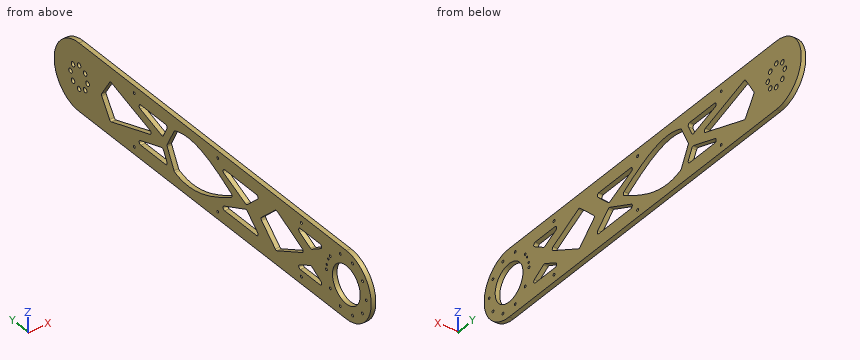
from build123d import *

# Parameters (mm, degrees)
SKETCH1_R           = 3.3
SKETCH1_R_2         = 1.7
SKETCH1_R_3         = 26
BOSS_EXTRUDE1_DEPTH = 6.35
CUT_EXTRUDE1_DEPTH  = 549.511460682
FILLET1_R           = 3
SKETCH4_R           = 1.75
CUT_EXTRUDE2_DEPTH  = 549.511460792
SKETCH5_R           = 1.2
CUT_EXTRUDE4_DEPTH  = 549.511460792


with BuildPart() as part:
    # Sketch1 → Boss-Extrude1 (new body)
    with BuildSketch(Plane(origin=(0, 0, 0), x_dir=(0, -1, 0), z_dir=(1, 0, 0))):
        with BuildLine():
            Line((0, 46.5), (500, 46.5))
            ThreePointArc((500, 46.5), (546.5, 0), (500, -46.5))
            Line((500, -46.5), (0, -46.5))
            ThreePointArc((0, -46.5), (-46.5, 0), (0, 46.5))
        make_face()
        with Locations(Location((-16, 0, 0), (0, 0, 90))):
            Circle(SKETCH1_R, mode=Mode.SUBTRACT)
        with Locations(Location((-11.313708499, 11.313708499, 0), (0, 0, 90))):
            Circle(SKETCH1_R, mode=Mode.SUBTRACT)
        with Locations(Location((0, 16, 0), (0, 0, 90))):
            Circle(SKETCH1_R, mode=Mode.SUBTRACT)
        with Locations(Location((11.313708499, 11.313708499, 0), (0, 0, 90))):
            Circle(SKETCH1_R, mode=Mode.SUBTRACT)
        with Locations(Location((16, 0, 0), (0, 0, 90))):
            Circle(SKETCH1_R, mode=Mode.SUBTRACT)
        with Locations(Location((11.313708499, -11.313708499, 0), (0, 0, 90))):
            Circle(SKETCH1_R, mode=Mode.SUBTRACT)
        with Locations(Location((537.25, 0, 0), (0, 0, 90))):
            Circle(SKETCH1_R_2, mode=Mode.SUBTRACT)
        with Locations(Location((530.13588304, -21.895000648, 0), (0, 0, 90))):
            Circle(SKETCH1_R_2, mode=Mode.SUBTRACT)
        with Locations(Location((511.51088304, -35.426855232, 0), (0, 0, 90))):
            Circle(SKETCH1_R_2, mode=Mode.SUBTRACT)
        with Locations(Location((488.48911696, -35.426855232, 0), (0, 0, 90))):
            Circle(SKETCH1_R_2, mode=Mode.SUBTRACT)
        with Locations(Location((469.86411696, -21.895000648, 0), (0, 0, 90))):
            Circle(SKETCH1_R_2, mode=Mode.SUBTRACT)
        with Locations(Location((462.75, 0, 0), (0, 0, 90))):
            Circle(SKETCH1_R_2, mode=Mode.SUBTRACT)
        with Locations(Location((469.86411696, 21.895000648, 0), (0, 0, 90))):
            Circle(SKETCH1_R_2, mode=Mode.SUBTRACT)
        with Locations(Location((488.48911696, 35.426855232, 0), (0, 0, 90))):
            Circle(SKETCH1_R_2, mode=Mode.SUBTRACT)
        with Locations(Location((511.51088304, 35.426855232, 0), (0, 0, 90))):
            Circle(SKETCH1_R_2, mode=Mode.SUBTRACT)
        with Locations(Location((530.13588304, 21.895000648, 0), (0, 0, 90))):
            Circle(SKETCH1_R_2, mode=Mode.SUBTRACT)
        with Locations(Location((500, 0, 0), (0, 0, 90))):
            Circle(SKETCH1_R_3, mode=Mode.SUBTRACT)
        with Locations(Location((0, -16, 0), (0, 0, 90))):
            Circle(SKETCH1_R, mode=Mode.SUBTRACT)
        with Locations(Location((-11.313708499, -11.313708499, 0), (0, 0, 90))):
            Circle(SKETCH1_R, mode=Mode.SUBTRACT)
    extrude(amount=BOSS_EXTRUDE1_DEPTH)

    # Sketch3 → Cut-Extrude1 (cut, through all)
    with BuildSketch(Plane(origin=(6.35, 0, 0), x_dir=(0, 0, -1), z_dir=(1, 0, 0))):
        Polygon((0, -422.848022722), (27.858212922, -368.632839363), (0, -339.139268075), (-27.858212922, -368.632839363), align=None)
        Polygon((0, -41.368651369), (-27.312924288, -58.435222232), (0, -141.248998295), (27.312924288, -58.435222232), align=None)
        Polygon((3, -313.189087212), (27.858212922, -339.506549748), (27.858212922, -258.646044282), align=None)
        Polygon((-27.858212922, -339.506549748), (-27.858212922, -258.646044282), (-3, -313.189087212), align=None)
        Polygon((-27.858212922, -401.452857349), (-11, -434.260816252), (-27.858212922, -461.481824785), align=None)
        Polygon((11, -434.260816252), (27.858212922, -461.481824785), (27.858212922, -401.452857349), align=None)
        with BuildLine():
            Line((0, -164.248853344), (-27.858212922, -178.200474573))
            add(Edge.make_bspline(
                [(-27.858212922, -178.200474573), (-43.7790539, -216.093343216), (-18.61661693, -258.276071598), (0, -289.085024731)],
                knots=[0, 0, 0, 0, 1, 1, 1, 1], degree=3))
            add(Edge.make_bspline(
                [(27.858212922, -178.200474573), (43.7790539, -216.093343216), (18.61661693, -258.276071598), (0, -289.085024731)],
                knots=[0, 0, 0, 0, 1, 1, 1, 1], degree=3))
            Line((27.858212922, -178.200474573), (0, -164.248853344))
        make_face()
        Polygon((7.5, -156.820958214), (27.312924288, -96.747453897), (27.312924288, -166.743432993), align=None)
        Polygon((-27.312924288, -96.747453897), (-27.312924288, -166.743432993), (-7.5, -156.820958214), align=None)
    extrude(amount=-CUT_EXTRUDE1_DEPTH, mode=Mode.SUBTRACT)

    # Fillet1
    fillet1_edges = [part.edges().sort_by_distance(p)[0] for p in [
        (3.175, -58.435222232, -27.312924288),
        (3.175, -41.368651369, 0),
        (3.175, -58.435222232, 27.312924288),
        (3.175, -141.248998295, 0),
        (3.175, -289.085024731, 0),
        (3.175, -164.248853344, 0),
        (3.175, -401.452857349, 27.858212922),
        (3.175, -434.260816252, 11),
        (3.175, -461.481824785, 27.858212922),
        (3.175, -461.481824785, -27.858212922),
        (3.175, -434.260816252, -11),
        (3.175, -401.452857349, -27.858212922),
        (3.175, -368.632839363, -27.858212922),
        (3.175, -339.139268075, 0),
        (3.175, -368.632839363, 27.858212922),
        (3.175, -422.848022722, 0),
        (3.175, -313.189087212, 3),
        (3.175, -339.506549748, 27.858212922),
        (3.175, -258.646044282, 27.858212922),
        (3.175, -178.200474573, -27.858212922),
        (3.175, -178.200474573, 27.858212922),
        (3.175, -339.506549748, -27.858212922),
        (3.175, -313.189087212, -3),
        (3.175, -258.646044282, -27.858212922),
        (3.175, -96.747453897, 27.312924288),
        (3.175, -166.743432993, 27.312924288),
        (3.175, -156.820958214, 7.5),
        (3.175, -166.743432993, -27.312924288),
        (3.175, -156.820958214, -7.5),
        (3.175, -96.747453897, -27.312924288),
    ]]
    fillet(fillet1_edges, radius=FILLET1_R)

    # Sketch4 → Cut-Extrude2 (cut, through all)
    with BuildSketch(Plane(origin=(6.35, 0, 0), x_dir=(0, 0, -1), z_dir=(1, 0, 0))):
        with Locations((-36.5, -103.175)):
            Circle(SKETCH4_R)
        with Locations(Location((36.5, -103.175, 0), (0, 0, 180))):
            Circle(SKETCH4_R)
        with Locations(Location((-36.5, -259.525, 0), (0, 0, 180))):
            Circle(SKETCH4_R)
        with Locations((36.5, -259.525)):
            Circle(SKETCH4_R)
        with Locations((-36.5, -415.875)):
            Circle(SKETCH4_R)
        with Locations(Location((36.5, -415.875, 0), (0, 0, 180))):
            Circle(SKETCH4_R)
    extrude(amount=-CUT_EXTRUDE2_DEPTH, mode=Mode.SUBTRACT)

    # Sketch5 → Cut-Extrude4 (cut, through all)
    with BuildSketch(Plane(origin=(6.35, 0, 0), x_dir=(0, 0, -1), z_dir=(1, 0, 0))):
        with Locations((-6.916110339, -463.343078174)):
            Circle(SKETCH5_R)
        with Locations((-15.951147244, -466.27873962)):
            Circle(SKETCH5_R)
    extrude(amount=-CUT_EXTRUDE4_DEPTH, mode=Mode.SUBTRACT)


solid = part.part
Here's how the part is built. I have some questions about the finished solid (model axes, mm). Coordinates: 2 decimals unless noted, no trailing zeros. Write each loop counter-clockwise with the first axis right and the second up, starting at its lowest first coordinate (ties: lowest second). Pieces come first, ordered by that corner, then holes.
Item 1: I want a section at C-C on y = -396. Write out the boundary of the cut face in (x, z), and give its area (3 significant figures).
Item 2: I want a section at B-B on x = 4. Count the separate pieces of the cut face and the enclosed holes in it, and give its area (3 significant figures).
Item 3: I want a section at A-A on y = -73. Write out the boundary of the cut face in (x, z), and give its area (3 significant figures).
Item 4: If I drill on line 1 (Z direction, x = 1.5, y = -469.5); line 2 (Y direction, x = 2.75, z = 36.5) (3 decimals); line 3 (Z direction, x = 0.5, y = 9), over which ranges is the centre line in solid material (lowest first)?
Findings below:
1. outline: (0, -46.5) - (6.35, -46.5) - (6.35, -13.8) - (0, -13.8) - close; (0, 13.8) - (6.35, 13.8) - (6.35, 46.5) - (0, 46.5) - close
1. area: 415 mm2
2. separate pieces: 1
2. enclosed holes: 36
2. area: 36,000 mm2
3. outline: (0, -46.5) - (6.35, -46.5) - (6.35, -22.51) - (0, -22.51) - close; (0, 22.51) - (6.35, 22.51) - (6.35, 46.5) - (0, 46.5) - close
3. area: 305 mm2
4. line 1: z = -46.5 to -23.56, -20.23 to 20.23, 23.56 to 46.5
4. line 2: y = -528.81 to -512.829, -510.192 to -489.808, -487.171 to -417.625, -414.125 to -261.275, -257.775 to -104.925, -101.425 to 28.81
4. line 3: z = -45.62 to -13.67, -8.96 to 8.96, 13.67 to 45.62
